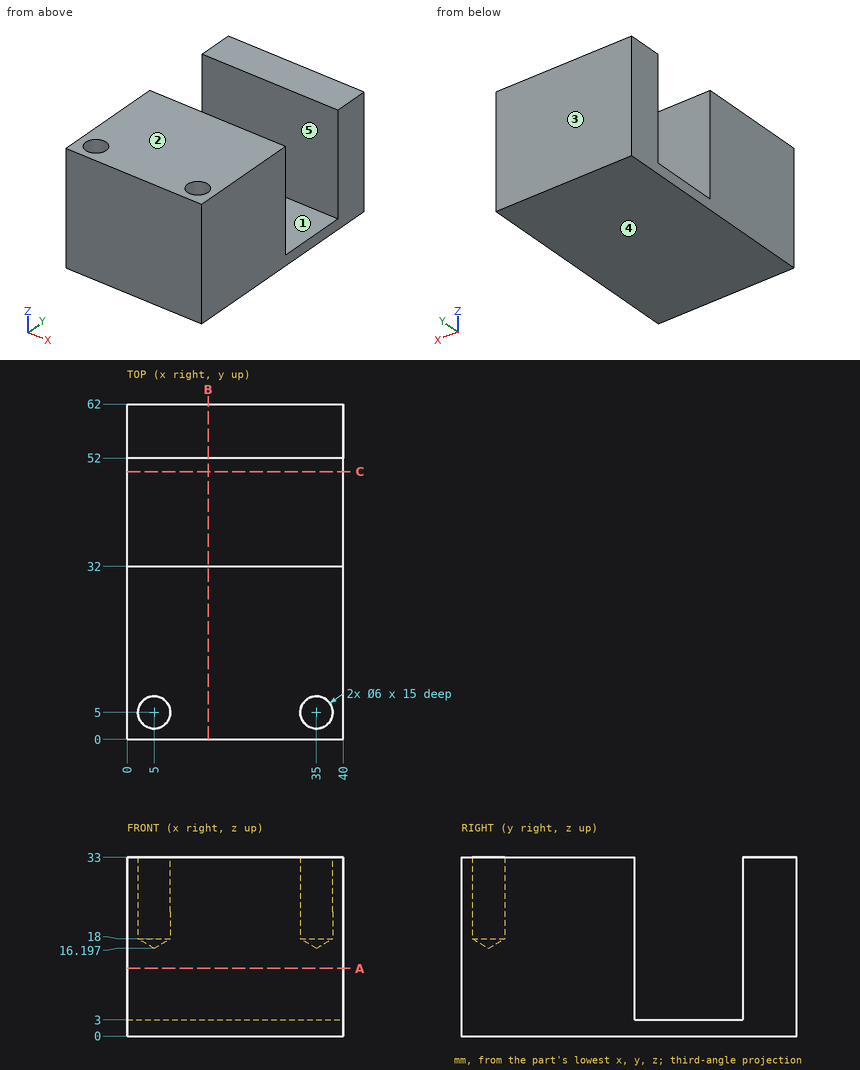
Verification items for this drawing (mm, ordinates from the low corner). A direction names the side the tool comes from. Give positions to 0.01 mm unless a question says otherwise; leave off trailing zeros. Write each loop counter-clockwise with the first axis right and the second up, starting at its lowest first coordinate (ties: lowest second). Pieces come first, ordered by that corner, then holes. Notation, with made-up numbers: (9.5, 86.5) - (25.5, 86.5) arc R31 cw to (25.5, 113.5) - close; hole circle Ø10 at (52.25, 70). An arc over 180 degrees is marked (long way). Answer as CSV lines item,"result". Start each with the question number.
1. Sectioned sample at B-B (x = 15). Record the boundary of the cut face in (y, z), then the cut area to 3 significant figures.
2. Draft check along Y on the marked faces 3, 4 and 5. Enter one of: pulls with the +Y half, pulls with the -Y half, needs draft (parallel to the pull), parting line crosses it, or undercut.
3. Sectioned sample at C-C (y = 49.5). Record the boundary of the cut face in (x, z).
4. Sectioned sample at A-A (z = 12.5). Record the boundary of the cut face in (x, y), then the cut area to 3 significant figures.
5. Depth check by flat-ended pin: pin 1 (5.5 mm diameter, centred on x = 5, y = 5, fed in from +Z); pin 2 (10 mm diameter, centred on x = 21, y = 40.5, fed in from +Z). Enter the tip coordinate at first touch or a pass-through.
6. Thickness scan on line 1 (Y direction, x = 5, z = 21.5); line 2 (Y direction, x = 9, z = 13); line 3 (X direction, y = 5, z = 29.5). Record the ranges inside material, lowest first.
7. Set-up check for the marked faces 1 and 2: record each of +Z, -Z, +X, -X, +Y, -Y from which the full face is reachable in a straight line by a thin tool's end or side.
Derived:
1,outline,"(0, 0) - (62, 0) - (62, 33) - (52, 33) - (52, 3) - (32, 3) - (32, 33) - (0, 33) - close"
1,area,"1,450 mm²"
2,face 3,"pulls with the +Y half"
2,face 4,"needs draft"
2,face 5,"undercut"
3,outline,"(0, 0) - (40, 0) - (40, 3) - (0, 3) - close"
4,outline,"(0, 0) - (40, 0) - (40, 32) - (0, 32) - close; (0, 52) - (40, 52) - (40, 62) - (0, 62) - close"
4,area,"1,680 mm²"
5,pin 1,"z = 17.85"
5,pin 2,"z = 3"
6,line 1,"0 to 2, 8 to 32, 52 to 62"
6,line 2,"0 to 32, 52 to 62"
6,line 3,"0 to 2, 8 to 32, 38 to 40"
7,face 1,"+Z, +X, -X"
7,face 2,"+Z, +X, -X, +Y, -Y"
